Verification items for the finished model (mm, model axes). A direction names the side the tool comes from. Coordinates: 2 decimals unless noted, no trailing zeros. Loops run counter-clockwise (first coordinate to the right, second up) from the corner with the lowest first, then second, coordinate; pieces in that order, holes last. Notation, with made-up numbers: (16.5, 81.25) -> (46.5, 81.25) arc R18 cw to (46.5, 109.25) -> close; hole circle Ø1 at (83, -25). An arc over 180 degrees is marked (long way). Write item = value, one per line.
```python
from build123d import *

# Parameters (mm, degrees)
SKETCH_1_W      = 16.4
SKETCH_1_H      = 11
EXTRUDE_1_DEPTH = 0.8
SKETCH_3_W      = 26.4
SKETCH_3_H      = 11
EXTRUDE_2_DEPTH = 0.8


with BuildPart() as part:
    # Эскиз1 → Бобышка-Вытянуть1 (new body)
    with BuildSketch(Plane(origin=(0, 0, 0), x_dir=(1, 0, 0), z_dir=(0, 1, 0))):
        Rectangle(SKETCH_1_W, SKETCH_1_H)
    extrude(amount=EXTRUDE_1_DEPTH)

    # Эскиз3 → Бобышка-Вытянуть2 (add)
    with BuildSketch(Plane.XZ):
        Rectangle(SKETCH_3_W, SKETCH_3_H)
    extrude(amount=EXTRUDE_2_DEPTH)


solid = part.part
```
1) Tool access check on faces 1 (the face through (0, -0.8, 0)), 2 (the face through (-11, 0, 0)), 3 (the face through (11, 0, 0)). Record the directions out of +Z, -Z, +X, -X, +Y, -Y that give a thin tool (end or side, any length) a straight path to the whole face; none if there is none.
Ans:
face_1 = +Z, -Z, +X, -X, -Y
face_2 = +Z, -Z, -X, +Y
face_3 = +Z, -Z, +X, +Y
2) Sectioned sample at B-B, the plane x = 10.25. Record the cut outline in (y, z).
Ans:
outline = (-0.8, -5.5) -> (0, -5.5) -> (0, 5.5) -> (-0.8, 5.5) -> close
3) Depth check by flat-ended pin: pin 1 Ø2.5 at (x, z) = (-9.5, -0.5) entering from +Y; pin 2 Ø0.6 at (y, z) = (0.5, -2) entering from +X. Enter the tip coordinate at first touch or a pass-through.
Ans:
pin_1 = 0
pin_2 = 8.2
4) Sectioned sample at A-A, the plane z = 2.25. Record the cut outline in (x, y).
Ans:
outline = (-13.2, -0.8) -> (13.2, -0.8) -> (13.2, 0) -> (8.2, 0) -> (8.2, 0.8) -> (-8.2, 0.8) -> (-8.2, 0) -> (-13.2, 0) -> close
5) Material ranges on line 1 (Y direction, x = -9, z = -4.5); line 2 (X direction, y = 0.3, z = -1.25), recorded low to high.
Ans:
line_1 = -0.8 to 0
line_2 = -8.2 to 8.2
6) Sectioned sample at C-C, the plane y = 0.3. Record the cut outline in (x, z).
Ans:
outline = (-8.2, -5.5) -> (8.2, -5.5) -> (8.2, 5.5) -> (-8.2, 5.5) -> close
